Check sheet for the modelled part. Datum: model origin and axes. Units: mm. A direction names the side the tool comes from. Give positions to 0.01 mm unless a question says otherwise; leave off trailing zeros. Loops run counter-clockwise (first coordinate to the right, second up) from the corner with the lowest first, then second, coordinate; pieces in that order, holes last. Notation, with made-up numbers: M -21,24.25 L -10,24.25 A20 ccw -10,28.25 Z; hole C 87.25,9.25 d8. An arc over 180 degrees is marked long. Write each question's results on one line, items separated by ' | '. Start each with the question number.
1. Sectioned sample at B-B on y = -7. Record the cut outline in (x, z).
2. Tool access check on faces 1 (the flat face through (24.5, -32, -7)), 2 (the flat face through (28.75, -32, -1)), 3 (the cylindrical face through (-0.02, -2.25, 5.04)). Record the directions out of +Z, -Z, +X, -X, +Y, -Y that give a thin tool (end or side, any length) a straight path to the whole face; none if there is none.
3. Draft check along X on faces 4 (the flat face through (36.5, -32, -1)), 5 (the flat face through (23.5, -31.5, -1)), 6 (the flat face through (32.25, -32, -1)). Enter one of: pulls with the +X half, pulls with the -X half, needs draft (parallel to the pull), parting line crosses it, or undercut.
4. Sectioned sample at C-C on y = -19.5. Record the cut outline in (x, z), and give its area (3 significant figures).
5. Material ranges on line 1 along Y through (x, z) = (9, 5.5); line 2 along X through (y, z) = (-26, 8.5); line 3 along Y through (x, z) = (2.5, 0.25), recorded low to high.
6. Go/stop test with flat-tipped pins: pin 1 (3.5 mm diameter, centred on y = -32, z = -4.5, fed in from -X); pin 2 (2.5 mm diameter, centred on x = -0.5, y = -9, fed in from -Z); pin 3 (6 mm diameter, centred on y = -18, z = -5, fed in from +X); pin 4 (11 mm diameter, centred on y = -15.5, z = 3, fed in from +X). Record where each tip stops, or that it passes through.
7. Sectioned sample at A-A on x = 30.5. Record the cut outline in (y, z).
8. Sectioned sample at D-D on z = -10.5. Record the cut outline in (x, y), and give its area (3 significant figures).
```python
from build123d import *

# Parameters (mm, degrees)
F4_W     = 3
F4_H     = 30
F4_W_2   = 12
F4_H_2   = 3
F5_DEPTH = 10
F0_DEPTH = 12
F2_DEPTH = 38.001
F7_DEPTH = 33.001
F3_SIZE  = 2


# Not quite as in the source:
# - a feature names something its author has since deleted; it is built from what else it names


with BuildPart() as f5:
    # F4 (on Top) → F5 (new body)
    with BuildSketch(Plane.XY):
        with Locations((0, -15)):
            Rectangle(F4_W, F4_H)
        Polygon((1.5, -30), (-1.5, -30), (-1.5, -33), (24.5, -33), (24.5, -30), align=None)
        with Locations((30.5, -31.5)):
            Rectangle(F4_W_2, F4_H_2)
    extrude(amount=F5_DEPTH)

    # F4 (on Top) → F0 (join)
    with BuildSketch(Plane.XY):
        with Locations((30.5, -31.5)):
            Rectangle(F4_W_2, F4_H_2)
    extrude(amount=-F0_DEPTH)

    # F1 (on face) → F2 (cut, through all)
    with BuildSketch(Plane(origin=(-1.5, 0, 0), x_dir=(0, -1, 0), z_dir=(-1, 0, 0))):
        with BuildLine():
            ThreePointArc((4, 3.25), (5.2374368671, 3.7625631329), (5.75, 5))
            ThreePointArc((5.75, 5), (5.2374368671, 6.2374368671), (4, 6.75))
            ThreePointArc((4, 6.75), (2.25, 5), (4, 3.25))
        make_face()
        with BuildLine():
            ThreePointArc((4, 6.75), (5.2374368671, 6.2374368671), (5.75, 5))
            ThreePointArc((5.75, 5), (5.2374368671, 3.7625631329), (4, 3.25))
            Line((4, 3.25), (10.5, 3.25))
            ThreePointArc((10.5, 3.25), (8.75, 5), (10.5, 6.75))
            Line((10.5, 6.75), (4, 6.75))
        make_face()
        with BuildLine():
            ThreePointArc((12.25, 5), (11.7374368671, 6.2374368671), (10.5, 6.75))
            ThreePointArc((10.5, 6.75), (8.75, 5), (10.5, 3.25))
            ThreePointArc((10.5, 3.25), (11.7374368671, 3.7625631329), (12.25, 5))
        make_face()
    extrude(amount=-F2_DEPTH, mode=Mode.SUBTRACT)

    # F6 (on face) → F7 (cut, through all)
    with BuildSketch(Plane.XZ.offset(33)):
        with BuildLine():
            ThreePointArc((28.75, -8), (30.5, -6.25), (32.25, -8))
            Line((32.25, -8), (32.25, 6))
            ThreePointArc((32.25, 6), (30.5, 4.25), (28.75, 6))
            Line((28.75, 6), (28.75, -8))
        make_face()
        with BuildLine():
            ThreePointArc((28.75, -8), (30.5, -9.75), (32.25, -8))
            ThreePointArc((32.25, -8), (30.5, -6.25), (28.75, -8))
        make_face()
        with BuildLine():
            ThreePointArc((28.75, 6), (30.5, 4.25), (32.25, 6))
            ThreePointArc((32.25, 6), (30.5, 7.75), (28.75, 6))
        make_face()
    extrude(amount=-F7_DEPTH, mode=Mode.SUBTRACT)

    # F3
    f3_edges = [f5.edges().sort_by_distance(p)[0] for p in [
        (1.5, -30, 5),
        (24.5, -31.5, 0),
    ]]
    chamfer(f3_edges, length=F3_SIZE)


solid = f5.part
```
Output values:
1) outline: M -1.5,0 L 1.5,0 L 1.5,3.25 L -1.5,3.25 Z; M -1.5,6.75 L 1.5,6.75 L 1.5,10 L -1.5,10 Z
2) face 1: -Z, -X, +Y, -Y | face 2: +Y, -Y | face 3: +X, -X
3) face 4: pulls with the +X half | face 5: pulls with the -X half | face 6: undercut
4) outline: M -1.5,0 L 1.5,0 L 1.5,10 L -1.5,10 Z | area: 30.0 mm2
5) line 1: -33 to -30 | line 2: -1.5 to 1.5 | line 3: -33 to -29
6) pin 1: x = 24.5 | pin 2: z = 0 | pin 3: through | pin 4: x = 1.5
7) outline: M -33,-12 L -30,-12 L -30,-9.75 L -33,-9.75 Z; M -33,7.75 L -30,7.75 L -30,10 L -33,10 Z
8) outline: M 24.5,-33 L 36.5,-33 L 36.5,-30 L 24.5,-30 Z | area: 36.0 mm2
